For this review, use the dimensioned drawing (mm, ordinates from the lowest corner) and the shaded views. A direction names the side the tool comes from. Give positions to 0.01 mm unless a question says otherwise; leave off trailing zeros. Write each loop counter-clockwise with the first axis right and the second up, starting at its lowest first coordinate (ties: lowest second). Pieces come first, ordered by that corner, then holes. Notation, with made-up numbers: M 62,44 L 85,44 A21 cw 85,49 Z; hole C -20,20.25 d4. An arc over 180 degrees is marked long. One line per item, written item: value. Start each with the question number.
Item 1: Tool access review of the marked faces 1 and 2: name each direction out of +Z, -Z, +X, -X, +Y, -Y from which nothing blocks a thin tool from reaching the whole face with its end or side.
Item 2: Consider section C-C, the plane y = 4.25. Write out the cut boundary in (x, z), and give its area (3 significant figures).
Item 3: Consider section A-A, the plane x = 38. Write out the cut boundary in (y, z).
Item 4: To check wall thickness, follow probe 1 along Y at (x, z) = (38.5, 6); probe 2 along Z at (x, y) = (57.5, 8); probe 3 along Z at (x, y) = (20, 6.75). State the ranges of each line that lie inside material, in increasing order.
Item 5: Clearance check with flat-ended pins moving along their axes: pin 1 Ø0.6 at (x, y) = (42.5, 8) entering from +Z; pin 2 Ø7 at (x, z) = (31.5, 23) entering from +Y; pin 3 Ø4.5 at (y, z) = (6, 18) entering from +X. State where each tip first meets the part, or that it passes through.
Item 6: Consider section D-D, the plane x = 8. Write out the cut boundary in (y, z).
Item 7: Consider section B-B, the plane z = 9. Write out the cut boundary in (x, y), and give its area (3 significant figures).
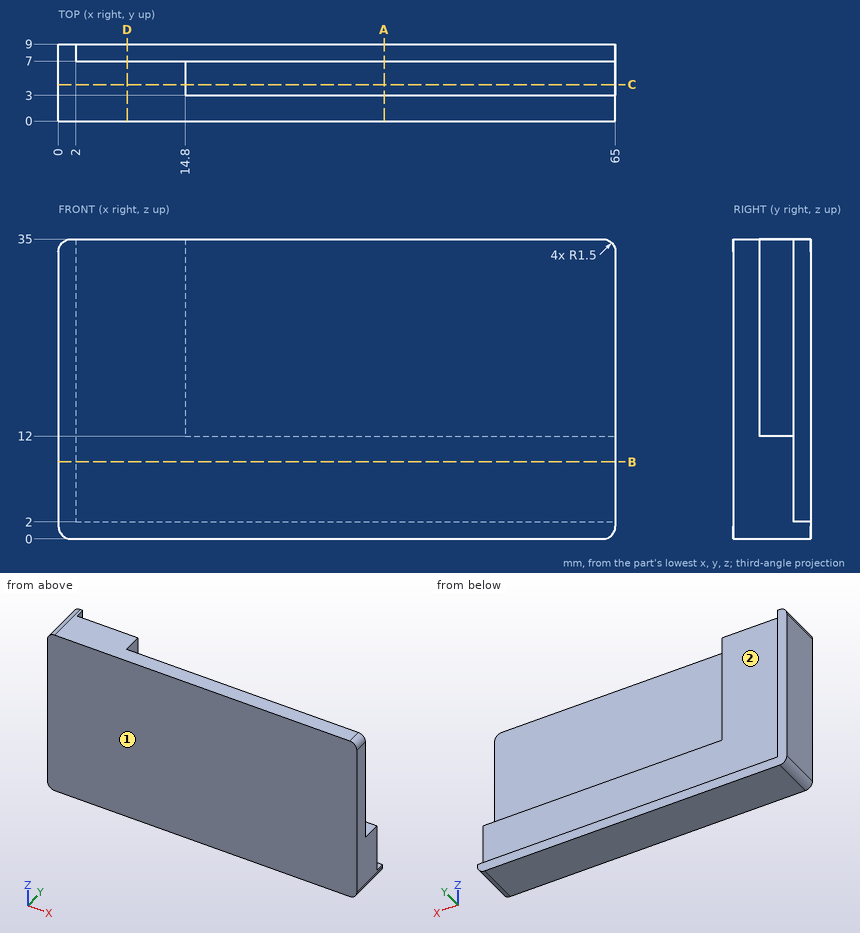
Model answer:
1. face 1: +Z, -Z, +X, -X, -Y
1. face 2: +Z, +X, +Y
2. outline: M 0,1.5 A1.5 ccw 1.5,0 L 63.5,0 A1.5 ccw 65,1.5 L 65,12 L 14.8,12 L 14.8,35 L 1.5,35 A1.5 ccw 0,33.5 Z
2. area: 1,120 mm2
3. outline: M 0,0 L 9,0 L 9,2 L 7,2 L 7,12 L 3,12 L 3,35 L 0,35 Z
4. probe 1: y = 0 to 7
4. probe 2: z = 0 to 2
4. probe 3: z = 0 to 12
5. pin 1: stops at z = 2
5. pin 2: stops at y = 3
5. pin 3: stops at x = 14.8
6. outline: M 0,0 L 9,0 L 9,2 L 7,2 L 7,35 L 0,35 Z
7. outline: M 0,0 L 65,0 L 65,7 L 2,7 L 2,9 L 0,9 Z
7. area: 459 mm2
